```python
from build123d import *

# Parameters (mm, degrees)
BOSS_EXTRUDE1_DEPTH = 12.7
CUT_EXTRUDE1_DEPTH  = 6.35
CHAMFER1_SIZE       = 6.35
SKETCH3_R           = 1.75
CUT_EXTRUDE2_DEPTH  = 6.35
SKETCH4_R           = 1.75
CUT_EXTRUDE3_DEPTH  = 4


with BuildPart() as part:
    # Sketch1 → Boss-Extrude1 (new body)
    with BuildSketch(Plane(origin=(0, 0, 0), x_dir=(1, 0, 0), z_dir=(0, 1, 0))):
        Polygon((-79.375, 0), (0, 0), (0, 79.375), (-3.175, 79.375), (-3.175, 77.7875), (-77.7875, 3.175), (-79.375, 3.175), align=None)
    extrude(amount=BOSS_EXTRUDE1_DEPTH)

    # Sketch2 → Cut-Extrude1 (cut)
    with BuildSketch(Plane(origin=(0, 12.7, 0), x_dir=(1, 0, 0), z_dir=(0, 1, 0))):
        Polygon((-73.297371939, 3.175), (-12.241098836, 3.175), (-3.175, 12.241098836), (-3.175, 73.297371939), align=None)
    extrude(amount=-CUT_EXTRUDE1_DEPTH, mode=Mode.SUBTRACT)

    # Chamfer1
    chamfer1_edges = [part.edges().sort_by_distance(p)[0] for p in [
        (-7.708049418, 6.35, -7.708049418),
    ]]
    chamfer(chamfer1_edges, length=CHAMFER1_SIZE - 0.0001)  # a hair under: the kernel refuses the full size

    # Sketch3 → Cut-Extrude2 (cut)
    with BuildSketch(Plane(origin=(0, 6.35, 0), x_dir=(1, 0, 0), z_dir=(0, 1, 0))):
        with Locations(Location((-44.460787159, 16.002, 0), (0, 0, 270))):
            Circle(SKETCH3_R)
        with Locations(Location((-15.875, 44.45, 0), (0, 0, 270))):
            Circle(SKETCH3_R)
    extrude(amount=-CUT_EXTRUDE2_DEPTH, mode=Mode.SUBTRACT)

    # Sketch4 → Cut-Extrude3 (cut)
    # profile 1 of 2: a face of its own
    with BuildSketch(Plane(origin=(0, 6.35, 0), x_dir=(1, 0, 0), z_dir=(0, 1, 0))):
        Polygon((-13.637767707, 40.575), (-11.400535414, 44.45), (-13.637767707, 48.325), (-18.112232293, 48.325), (-20.349464586, 44.45), (-18.112232293, 40.575), align=None)
        with Locations(Location((-15.875, 44.45, 0), (0, 0, 270))):
            Circle(SKETCH4_R, mode=Mode.SUBTRACT)
    # profile 2 of 2: a face of its own
    with BuildSketch(Plane(origin=(0, 6.35, 0), x_dir=(1, 0, 0), z_dir=(0, 1, 0))):
        Polygon((-39.986322573, 16.002), (-42.223554866, 19.877), (-46.698019452, 19.877), (-48.935251745, 16.002), (-46.698019452, 12.127), (-42.223554866, 12.127), align=None)
        with Locations(Location((-44.460787159, 16.002, 0), (0, 0, 270))):
            Circle(SKETCH4_R, mode=Mode.SUBTRACT)
    extrude(amount=-CUT_EXTRUDE3_DEPTH, mode=Mode.SUBTRACT)


solid = part.part
```
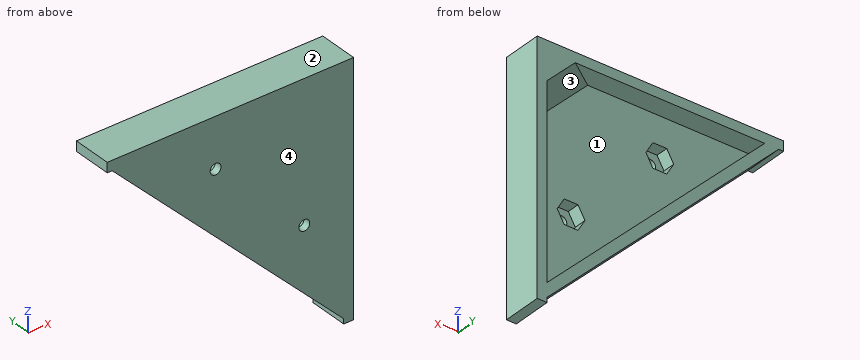
Could you check a few things on this model? Use its own coordinates, in mm. Face numbers are marked on the shaded views. Coordinates: 2 decimals unless noted, no trailing zeros. Write each loop counter-clockwise with the first axis right and the second up, starting at its lowest first coordinate (ties: lowest second). Pieces come first, ordered by that corner, then holes. Notation, with made-up numbers: M 6.5,0 L 12.5,0 A19 cw 12.5,23 Z; hole C 8,21.5 d2. An arc over 180 degrees is marked long. Answer as CSV lines item,"result". Start each with the question number.
1) I want a section at B-B, the plane y = 9. Please give me the cut outline in (x, z) (1 decimal).
2) We'd pull the mould along Z, two halves only. Please class the marked faces 1, 2, 3 and 4: +Z half, -Z half, draft (parallel to the pull), parting line (faces both ways), or undercut.
3) For P1, Ø1.2, axis at x = -44, y = 4, coming from the -Z side; P2, Ø4, axis at y = 4, z = -27, coming from the -X side; P3, Ø1.3, axis at x = -78.5, y = 7, coming from the -Z side (3 decimals); P4, Ø3, axis at x = -15.875, z = -44.45, coming from the +Y side, each with a flat end and sliding along its axis, tell me the tip position at first contact or that it passes through.
4) Please list where these lines run through material, in increasing order: line 1 (Y direction, x = -36, z = -12); line 2 (Z direction, x = -18, y = 11.25) (1 decimal); line 3 (X direction, y = 3.25, z = -48). Write a range as from..to.
5) I want a section at A-A, the plane y = 3.5. Give the number of separate pieces and of enclosed holes in the cut face, and give its area (3 significant figures).
Data:
1,outline,"M -79.4,-3.2 L -77.8,-3.2 L -3.2,-77.8 L -3.2,-79.4 L 0,-79.4 L 0,0 L -79.4,0 Z; hole M -73.3,-3.2 L -3.2,-73.3 L -3.2,-17.5 L -17.5,-3.2 Z"
2,face 1,"undercut"
2,face 2,"+Z half"
2,face 3,"undercut"
2,face 4,"draft"
3,P1,"stops at z = -37.56"
3,P2,"stops at x = -55.96"
3,P3,"stops at z = -3.175"
3,P4,"passes through"
4,line 1,"y = 0..6.35"
4,line 2,"z = -63..-58.5, -3.2..0"
4,line 3,"x = -32.96..-18.3, -13.45..0"
5,separate pieces,"1"
5,enclosed holes,"2"
5,area,"3,170 mm^2"
